Geometry: final body of the model. Coordinates: model frame, mm. Give positions to 0.01 mm unless a question says otherwise; leave off trailing zeros. Write each loop counter-clockwise with the first axis right and the second up, starting at its lowest first coordinate (ties: lowest second). Pieces come first, ordered by that corner, then holes. Notation, with made-up numbers: M 46,27.25 L 86,27.25 A12 ccw 86,38.25 Z; hole C -8.5,28 d11. An arc over 180 degrees is marked long. Answer as a JSON object with one key per item and string values.
from build123d import *

# Parameters (mm, degrees)
SKETCH1_R             = 4.7625
BOSS_EXTRUDE1_DEPTH   = 4.37
FILLET1_R             = 5
M3X0_5_TAPPED_HOLE1_D = 2.5


with BuildPart() as part:
    # Sketch1 → Boss-Extrude1 (new body)
    with BuildSketch(Plane(origin=(0, 0, 0), x_dir=(0, 0, -1), z_dir=(1, 0, 0))):
        with BuildLine():
            Line((0, 7.5), (12, 7.5))
            Line((12, 7.5), (12, -7.5))
            Line((12, -7.5), (0, -7.5))
            ThreePointArc((0, -7.5), (-7.5, 0), (0, 7.5))
        make_face()
        Circle(SKETCH1_R, mode=Mode.SUBTRACT)
    extrude(amount=BOSS_EXTRUDE1_DEPTH)

    # Fillet1
    fillet1_edges = [part.edges().sort_by_distance(p)[0] for p in [
        (2.185, -7.5, -12),
        (2.185, 7.5, -12),
    ]]
    fillet(fillet1_edges, radius=FILLET1_R)

    # M3x0.5 Tapped Hole1 (through all)
    with Locations(Plane.ZY):
        with Locations((-6.905099565, 4), (-6.905099565, -4)):
            Hole(M3X0_5_TAPPED_HOLE1_D / 2)


solid = part.part
1) Cut plane B-B on x = 2.4. Give the number of separate pieces and of enclosed holes in the cut face, and give its area (3 significant figures).
Geometry check:
{"separate pieces": "1", "enclosed holes": "3", "area": "177 mm2"}
2) Contact query for a flat-ended pin moving along its axis: P1, Ø2, axis at y = 4, z = -6.91, coming from the -X side. Output: stop coordinate, or through.
Geometry check:
{"P1": "passes through"}
3) Cut plane D-D on y = -4. Return loops of the section in (x, z), and give its area (3 significant figures).
Geometry check:
{"outline": "M 0,-11.77 L 4.37,-11.77 L 4.37,-8.16 L 0,-8.16 Z; M 0,-5.66 L 4.37,-5.66 L 4.37,-2.58 L 0,-2.58 Z; M 0,2.58 L 4.37,2.58 L 4.37,6.34 L 0,6.34 Z", "area": "45.6 mm2"}
4) Pull-direction query (Y, two-part tool) for faces 1 (the flat face through (2, 7.5, -3)), 2 (the cylindrical face through (2.216, 3.239, -5.913)), 3 (the flat face through (2, 0, -12)); classes: pulls with the +Y half, pulls with the -Y half, needs draft (parallel to the pull), parting line crosses it, or undercut.
Geometry check:
{"face 1": "pulls with the +Y half", "face 2": "undercut", "face 3": "needs draft"}
5) Cut plane C-C on y = -1.5. Return loops of the section in (x, z), and give its area (3 significant figures).
Geometry check:
{"outline": "M 0,-12 L 4.37,-12 L 4.37,-4.52 L 0,-4.52 Z; M 0,4.52 L 4.37,4.52 L 4.37,7.35 L 0,7.35 Z", "area": "45.0 mm2"}
6) Line query: line 1 (Y direction, x = 3.95, z = -6); line 2 (Z direction, x = 3.8, y = 3.25); line 3 (Z direction, x = 3.45, y = -3.75). Output: solid intervals per line, ascending. Write a range as from..to.
Geometry check:
{"line 1": "y = -7.5..-4.86, -3.14..3.14, 4.86..7.5", "line 2": "z = -11.94..-7.91, -5.91..-3.48, 3.48..6.76", "line 3": "z = -11.84..-8.13, -5.68..-2.94, 2.94..6.5"}
7) Cut plane A-A on z = -4.5. Return loops of the section in (x, y).
Geometry check:
{"outline": "M 0,-7.5 L 4.37,-7.5 L 4.37,-1.56 L 0,-1.56 Z; M 0,1.56 L 4.37,1.56 L 4.37,7.5 L 0,7.5 Z"}
